Work out the finished part from the listing and answer in its coordinate system (mm). A direction names the side the tool comes from. Coordinates: 2 decimals unless noted, no trailing zeros. Order: outer loops, then holes, each group sorted by start corner. A loop starts at its lowest first (then second) coordinate and runs counter-clockwise, first axis right, second up. Notation, with made-up numbers: M 0,41 L 21,41 A30 ccw 21,73 Z; hole C 30.5,67.5 d8. An arc over 180 degrees is marked long. Use a Markdown table: item, result. Add a question column.
from build123d import *

# Parameters (mm, degrees)
BOSS_EXTRUDE2_DEPTH = 3
BOSS_EXTRUDE3_DEPTH = 33.5
CUT_EXTRUDE1_DEPTH  = 3


with BuildPart() as part:
    # Sketch1 → Boss-Extrude2 (new body)
    with BuildSketch(Plane.XY):
        with BuildLine():
            ThreePointArc((-37.5, 24), (-61.5, 0), (-37.5, -24))
            Line((-37.5, -24), (39.664725273, -23.90217489))
            ThreePointArc((39.664725273, -23.90217489), (61.475531249, 1.083467265), (37.5, 24))
            Line((37.5, 24), (-37.5, 24))
        make_face()
    extrude(amount=BOSS_EXTRUDE2_DEPTH)

    # Sketch3 → Boss-Extrude3 (add)
    with BuildSketch(Plane.XY.offset(3)):
        with BuildLine():
            ThreePointArc((-37.5, 24), (-61.5, 0), (-37.5, -24))
            Line((-37.5, -24), (39.664725273, -23.90217489))
            ThreePointArc((39.664725273, -23.90217489), (61.475531249, 1.083467265), (37.5, 24))
            Line((37.5, 24), (-37.5, 24))
        make_face()
        with BuildLine():
            ThreePointArc((-37.5, -21), (-58.5, 0), (-37.5, 21))
            Line((-37.5, 21), (37.5, 21))
            ThreePointArc((37.5, 21), (58.5, 0), (37.5, -21))
            Line((37.5, -21), (-37.5, -21))
        make_face(mode=Mode.SUBTRACT)
    extrude(amount=BOSS_EXTRUDE3_DEPTH)

    # Sketch4 → Cut-Extrude1 (cut)
    with BuildSketch(Plane(origin=(0, 0, 0), x_dir=(-1, 0, 0), z_dir=(0, 0, -1))):
        with BuildLine():
            ThreePointArc((-37.5, 18), (-55.5, 0), (-37.5, -18))
            Line((-37.5, -18), (37.5, -18))
            ThreePointArc((37.5, -18), (55.5, 0), (37.5, 18))
            Line((37.5, 18), (-37.5, 18))
        make_face()
    extrude(amount=-CUT_EXTRUDE1_DEPTH, mode=Mode.SUBTRACT)


solid = part.part
(1) Which of the six approach directions +Z, -Z, +X, -X, +Y, -Y give full straight-line access (tool end or side, diameter ignored) to faces 1 (the cylindrical face through (-55.496, -0.396, 1.479)), 2 (the flat face through (-0.3, 21.4, 36.5)), 3 (the flat face through (-1, 21, 20))?
(2) Given P1, Ø2.5, axis at x = -5, z = 2, coming from the -Y side; P2, Ø21, axis at x = -25, y = 8, coming from the +Z side; P3, Ø8, axis at y = 16, z = 31.5, coming from the -X side, each flat-ended and moving along its own axis, determine where each tip first touches the part or whether it passes through.
(3) Straight lines are drawn through the part: line 1 (Y direction, x = 18.5, z = 22); line 2 (X direction, y = 0, z = 30.5); line 3 (Y direction, x = -20.5, z = 31.5). For each, find the intervals that lie inside material, in ascending order.
(4) A cutting plane is placed at A-A on z = 11. Write down the section's boundary in (x, y), plus the area to 3 significant figures.
(5) A cutting plane is placed at C-C on x = -5. Write down the section's boundary in (y, z), plus the area to 3 significant figures.
(6) A cutting plane is placed at B-B on y = 0. Write down the section's boundary in (x, z), plus the area to 3 significant figures.
(7) The mould has two halves that part along X. Classify faces 4 (the cylindrical face through (-61.494, 0.528, 17.994)), 5 (the cylindrical face through (61.493, 0.571, 17.994)), 6 (the flat face through (0, -19, 0)), 7 (the flat face through (1, -21, 20)): pulls with the +X half, pulls with the -X half, needs draft (parallel to the pull), parting line crosses it, or undercut.
From the geometry:
| question | item | result |
|---|---|---|
| 1 | face 1 | +Z, -Z |
| 1 | face 2 | +Z, +X, -X, +Y, -Y |
| 1 | face 3 | +Z |
| 2 | P1 | stops at y = -23.96 |
| 2 | P2 | stops at z = 3 |
| 2 | P3 | stops at x = -58.28 |
| 3 | line 1 | y = -23.93 to -21, 21 to 24 |
| 3 | line 2 | x = -61.5 to -58.5, 58.5 to 61.5 |
| 3 | line 3 | y = -23.98 to -21, 21 to 24 |
| 4 | outline | M -37.5,-24 L 39.66,-23.9 A24 ccw 37.5,24 L -37.5,24 A24 ccw Z; hole M -37.5,-21 L 37.5,-21 A21 ccw 37.5,21 L -37.5,21 A21 ccw Z |
| 4 | area | 870 mm2 |
| 5 | outline | M -23.96,0 L -18,0 L -18,3 L -21,3 L -21,36.5 L -23.96,36.5 Z; M 18,0 L 24,0 L 24,36.5 L 21,36.5 L 21,3 L 18,3 Z |
| 5 | area | 235 mm2 |
| 6 | outline | M -61.5,0 L -55.5,0 L -55.5,3 L -58.5,3 L -58.5,36.5 L -61.5,36.5 Z; M 55.5,0 L 61.5,0 L 61.5,36.5 L 58.5,36.5 L 58.5,3 L 55.5,3 Z |
| 6 | area | 237 mm2 |
| 7 | face 4 | pulls with the -X half |
| 7 | face 5 | pulls with the +X half |
| 7 | face 6 | needs draft |
| 7 | face 7 | undercut |
